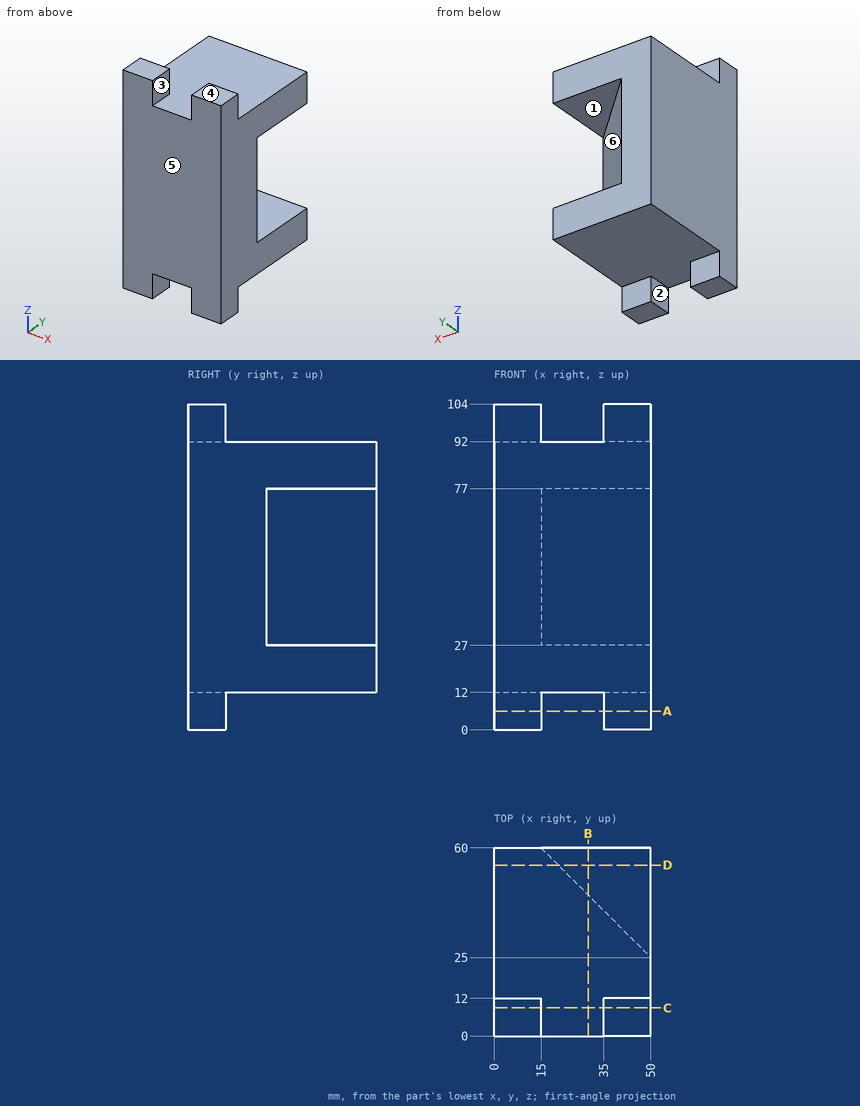
Can you work these out from the drawing? Everything is in mm from the part's minimum corner. A direction names the side the tool comes from. Round coordinates to 2 decimals unless told otherwise and drop trailing zeros. Write each loop counter-clockwise with the first axis right and the second up, starting at its lowest first coordinate (ties: lowest second). Pieces come first, ordered by that corner, then holes.
1. If we mould it in two halves opening along Z, with no side actions, what happens to the marked faces 4, 5 and 6? For each: released by +Z, released by -Z, zero draft, split by the parting line, or undercut.
2. Suppose I cut it at A-A (z = 6). List the corners of the cut face in (x, y) for me.
3. I need wall thicknesses on L1, parallel to Z at x = 24, y = 51.5; L2, parallel to X at y = 3.5, z = 9; L3, parallel to Z at x = 20.5, y = 19.5. Which ranges of each line are inside material? Lowest first, please.
4. Will these pins go through, and if not, where does the flat tip stop? pin 1 Ø17.5 at (x, y) = (28.5, 47.5) entering from -Z; pin 2 Ø13 at (x, z) = (41, 99) entering from +Y; pin 3 Ø6 at (x, y) = (37, 53) entering from +Z.
5. For the marked faces 1, 2 and 3, which set-ups out of +Z, -Z, +X, -X, +Y, -Y let a thin tool reach every point of the face, with its end or its side?
6. Suppose I cut it at C-C (y = 9). List the corners of the cut face in (x, z) for me, and give its area (3 significant figures).
7. Suppose I cut it at D-D (y = 54.5). List the corners of the cut face in (x, z) for me.
8. Suppose I cut it at B-B (x = 30). List the corners of the cut face in (y, z) for me, and give its area (3 significant figures).
Answer sheet:
1. face 4: released by +Z
1. face 5: zero draft
1. face 6: undercut
2. outline: (0, 0) - (15, 0) - (15, 12) - (0, 12) - close; (35, 0) - (50, 0) - (50, 12) - (35, 12) - close
3. L1: z = 12 to 27, 77 to 92
3. L2: x = 0 to 15, 35 to 50
3. L3: z = 12 to 92
4. pin 1: stops at z = 12
4. pin 2: stops at y = 12
4. pin 3: stops at z = 92
5. face 1: +X, +Y
5. face 2: -Z, +Y, -Y
5. face 3: +Z, +Y, -Y
6. outline: (0, 0) - (15, 0) - (15, 12) - (35, 12) - (35, 0) - (50, 0) - (50, 104) - (35, 104) - (35, 92) - (15, 92) - (15, 104) - (0, 104) - close
6. area: 4,720 mm2
7. outline: (0, 12) - (50, 12) - (50, 27) - (20.5, 27) - (20.5, 77) - (50, 77) - (50, 92) - (0, 92) - close
8. outline: (0, 12) - (60, 12) - (60, 27) - (45, 27) - (45, 77) - (60, 77) - (60, 92) - (0, 92) - close
8. area: 4,050 mm2
